Model file for the job. Use its own axes, mm. Round coordinates to 2 decimals unless told otherwise and drop trailing zeros. Order: outer loops, then holes, each group sorted by start corner. A loop starts at its lowest first (then second) coordinate and runs counter-clockwise, first axis right, second up. Notation, with made-up numbers: (7, 46.25) - (25, 46.25) arc R32 ccw to (25, 72.25) - close; hole circle Ø4 at (70.25, 28.25). An arc over 180 degrees is marked (long way). Answer as CSV lines item,"result". Start each with the question number.
1. Band-saw the part on B-B on y = -14. List the corners of the cut face in (x, z), then the cut area to 3 significant figures.
2. Pin check, flat tips, straight feed: pin 1 Ø3 at (y, z) = (-14, 1) entering from +X; pin 2 Ø3 at (y, z) = (27, 2) entering from -X; pin 3 Ø11.5 at (x, y) = (83.53, 12.7) entering from +Z; pin 4 Ø2 at (x, z) = (148.5, 4.5) entering from -Y. Stop position of each tip, or through.
3. Band-saw the part on C-C on x = 18. List the corners of the cut face in (y, z).
4. Band-saw the part on A-A on z = 4.75. State how many separate pieces and enclosed holes the cut face has, then the cut area to 3 significant figures.
5. Wall check: line 1 along Y through (x, z) = (130.5, 5.75); line 2 along X through (y, z) = (9.5, 6); line 3 along Y through (x, z) = (54, 4.75). Give the ranges that are in metal, low to high. Write a range as [from, to].
Autodesk Inventor part; units mm, degrees
ref_plane "YZ Plane" through (0, 0, 0) normal (1, 0, 0) x (0, 1, 0)
ref_plane "XZ Plane" through (0, 0, 0) normal (0, 1, 0) x (-1, 0, 0)
ref_plane "XY Plane" through (0, 0, 0) normal (0, 0, 1) x (1, 0, 0)
sketch "Sketch1" plane through (0, 0, 0) normal (0, 0, 1) x (1, 0, 0)
  line L0 (0, 0) -> (130.048, 0)
  line L1 (87.9024, 12.7) -> (7.3323, 12.7)
  line L2 (87.9024, 12.7) -> (130.048, 12.7)
  line L3 (130.048, 12.7) -> (130.048, 0)
  line L4 (130.048, -31.75) -> (142.748, -31.75)
  line L5 (130.048, -31.75) -> (148.3789, 0)
  line L6 (142.748, -31.75) -> (168.4112, 12.7)
  line L7 (148.3789, 0) -> (130.048, 0)
  line L8 (130.048, 12.7) -> (168.4112, 12.7)
  line L9 (7.3323, 12.7) -> (-3.6662, 19.05)
  line L10 (-3.6662, 19.05) -> (-10.9985, 6.35)
  line L11 (-10.9985, 6.35) -> (0, 0)
  dimension "d4" = 130.048
  dimension "d7" = 31.75
  dimension "d8" = 12.7
  dimension "d9" = 60
  dimension "d10" = 60
  dimension "d11" = 12.7
  dimension "d14" = 12.7
  dimension "d15" = 10.9985
  dimension "d16" = 14.6647
  dimension "d17" = 150
  dimension "d18" = 150
extrude "Extrusion1" add sketch "Sketch1" along normal blind 6.35
sketch "Sketch2" plane through (0, 0, 6.35) normal (0, 0, 1) x (1, 0, 0)
  line L0 (168.4112, 12.7) -> (7.3323, 12.7)
  line L1 (-10.9985, 6.35) -> (0, 0)
  line L2 (7.3323, 12.7) -> (20.426, 35.379)
  line L3 (20.426, 35.379) -> (168.4112, 12.7)
  dimension "d19" = 26.1874
extrude "Extrusion2" add sketch "Sketch2" against normal blind 6.35
fillet "Fillet1" radius 3.175 1 edges at (168.4112, 12.7, 3.175)
fillet "Fillet2" radius 3.175 1 edges at (142.748, -31.75, 3.175)
sketch "Sketch3" plane through (0, 0, 6.35) normal (0, 0, 1) x (1, 0, 0)
  circle A0 centre (32.7323, 12.7) radius 6.35
  circle A1 centre (58.1323, 12.7) radius 6.35
  circle A2 centre (83.5323, 12.7) radius 6.35
  dimension "d26" = 12.7
  dimension "d28" = 12.7
  dimension "d30" = 12.7
extrude "Extrusion3" cut sketch "Sketch3" against normal blind 6.35
fillet "Fillet4" radius 6.35 1 edges at (148.3789, 0, 3.175)
properties part number "hook" material "Steel"
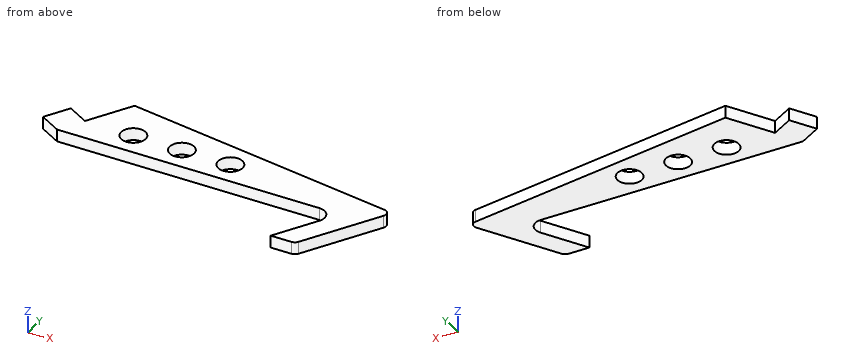
Reply:
1,outline,"(140.3, 0) - (153, 0) - (153, 6.35) - (140.3, 6.35) - close"
1,area,"80.6 mm2"
2,pin 1,"stops at x = 153.86"
2,pin 2,"stops at x = 14.72"
2,pin 3,"passes through"
2,pin 4,"stops at y = -23.52"
3,outline,"(0, 0) - (31.18, 0) - (31.18, 6.35) - (0, 6.35) - close"
4,separate pieces,"1"
4,enclosed holes,"3"
4,area,"4,100 mm2"
5,line 1,"y = [-31.75, -30.97], [0, 18.51]"
5,line 2,"x = [-9.18, 27.25], [38.22, 52.65], [63.62, 78.05], [89.02, 166.42]"
5,line 3,"y = [0, 7.88], [17.52, 30.23]"
